from build123d import *

# Parameters (mm, degrees)
F0_R           = 3.5
F1_DEPTH       = 3
F3_DEPTH       = 20
F5_D           = 3.3
F5_CSINK_D     = 8.96
F5_CSINK_ANGLE = 90


with BuildPart() as f1:
    # F0 (on Front) → F1 (new body)
    with BuildSketch(Plane.XZ):
        with BuildLine():
            Line((0, 19), (0, 0))
            Line((0, 0), (38, 0))
            Line((38, 0), (38, 4))
            Line((38, 4), (18, 4))
            Line((18, 4), (18, 19))
            ThreePointArc((18, 19), (9, 10), (0, 19))
        make_face()
        with BuildLine():
            ThreePointArc((18, 19), (9, 28), (0, 19))
            ThreePointArc((0, 19), (9, 10), (18, 19))
        make_face()
        with Locations((9, 19)):
            Circle(F0_R, mode=Mode.SUBTRACT)
    extrude(amount=F1_DEPTH)

    # F2 (on face) → F3 (join)
    with BuildSketch(Plane.XZ.offset(3)):
        Polygon((0, 0), (38, 0), (38, 4), (18, 4), (0, 4), align=None)
    extrude(amount=F3_DEPTH)

    # F5 (through all)
    with Locations(Plane.XY.offset(4)):
        with Locations((19, -11.5)):
            CounterSinkHole(F5_D / 2, F5_CSINK_D / 2, counter_sink_angle=F5_CSINK_ANGLE)


solid = f1.part
Verification items for the finished model (mm, model axes). A direction names the side the tool comes from. Give positions to 0.01 mm unless a question says otherwise; leave off trailing zeros. Order: outer loops, then holes, each group sorted by start corner. A loop starts at its lowest first (then second) coordinate and runs counter-clockwise, first axis right, second up. Notation, with made-up numbers: M 71.25,-32.5 L 103.25,-32.5 A13 ccw 103.25,-24.5 Z; hole C 9.5,15 d1. An arc over 180 degrees is marked long. Answer as a JSON object with one key per item and string values. Group by question number.
1) Scan lines: line 1 along Z through (x, y) = (9, -1.65); line 2 along Y through (x, z) = (19, 0.6); line 3 along Y through (x, z) = (17, 10.75). Record each from-to range of solid material in increasing order. Write a range as [from, to].
2) Cross-section at C-C (y = -2.5). Enter the section's corners in (x, z), then the cut area to 3 significant figures.
3) Mould release check, pull along Z, two halves, no side actions. Record for faces 3 (the face through (6.42, -1.479, 21.365)), 4 (the face through (17.349, -12.185, 1.307)), 5 (the face through (9, -3, 14)): released by +Z, released by -Z, zero draft, split by the parting line, or undercut.
4) Access from +Z, -Z, +X, -X, +Y, -Y to the whole of each face (thin tool, end or side, straight path). Record for faces 1 (the face through (19, -23, 2)), 2 (the face through (18, -1, 11)).
5) Cross-section at B-B (x = 19). Enter the section's corners in (y, z).
6) Cross-section at D-D (z = 21.75). Enter the section's corners in (x, y), then the cut area to 3 significant figures.
7) Cross-section at A-A (y = -11.5). Enter the section's corners in (x, z), then the cut area to 3 significant figures.
8) Depth check by flat-ended pin: pin 1 Ø1 at (x, y) = (26, -10) entering from -Z; pin 2 Ø5.5 at (x, z) = (9, 19) entering from +Y; pin 3 Ø2.5 at (y, z) = (-1.5, 9.5) entering from +X; pin 4 Ø4 at (y, z) = (-4.5, 23.5) entering from +X. Enter the tip coordinate at first touch or a pass-through.
Result sheet:
{
 "1": {"line 1": "z = [0, 15.5], [22.5, 28]", "line 2": "y = [-23, -13.15], [-9.85, 0]", "line 3": "y = [-3, 0]"},
 "2": {"outline": "M 0,0 L 38,0 L 38,4 L 18,4 L 18,19 A9 ccw 0,19 Z; hole C 9,19 d7", "area": "511 mm2"},
 "3": {"face 3": "undercut", "face 4": "released by +Z", "face 5": "zero draft"},
 "4": {"face 1": "+Z, -Z, +X, -X, -Y", "face 2": "+Z, +X, +Y, -Y"},
 "5": {"outline": "M -23,0 L -13.15,0 L -13.15,1.17 L -15.98,4 L -23,4 Z; M -9.85,0 L 0,0 L 0,4 L -7.02,4 L -9.85,1.17 Z"},
 "6": {"outline": "M 0.43,-3 L 6.83,-3 L 6.83,0 L 0.43,0 Z; M 11.17,-3 L 17.57,-3 L 17.57,0 L 11.17,0 Z", "area": "38.4 mm2"},
 "7": {"outline": "M 0,0 L 17.35,0 L 17.35,1.17 L 14.52,4 L 0,4 Z; M 20.65,0 L 38,0 L 38,4 L 23.48,4 L 20.65,1.17 Z", "area": "131 mm2"},
 "8": {"pin 1": "stops at z = 0", "pin 2": "passes through", "pin 3": "stops at x = 18", "pin 4": "stops at x = 17.42"}
}
